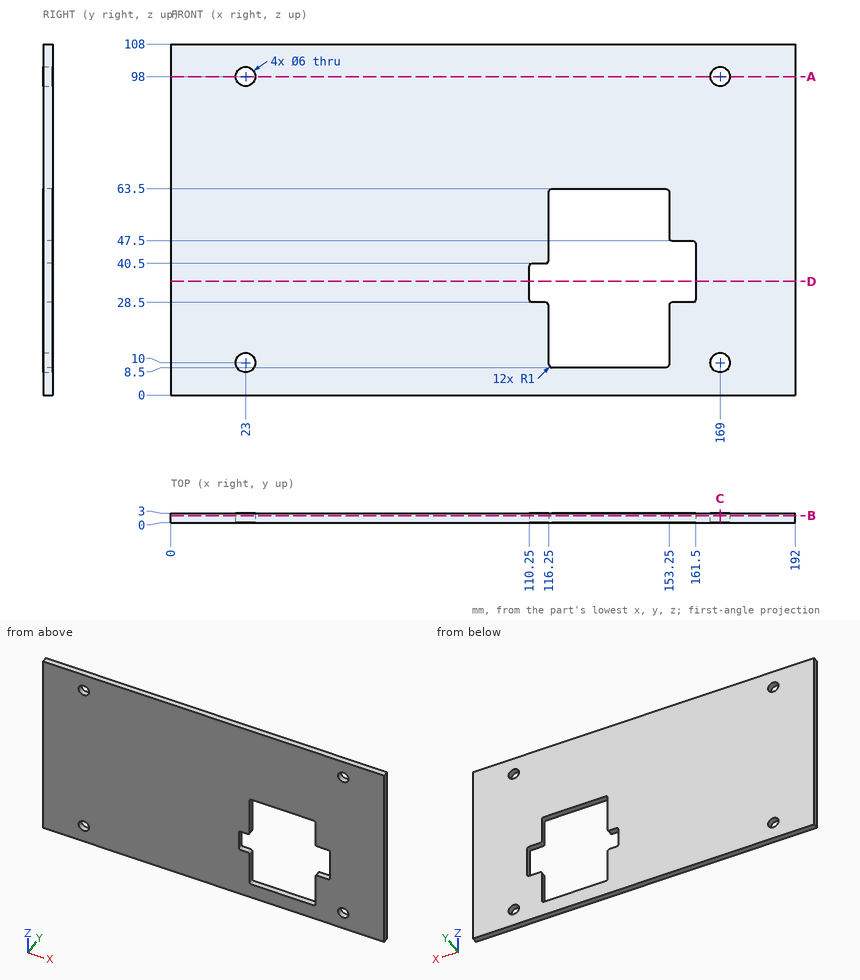
Check sheet for the drawn part. Datum: minimum x, y, z corner. Units: mm. Round coordinates to 2 decimals unless told otherwise and drop trailing zeros. Write each loop counter-clockwise with the first axis right and the second up, starting at its lowest first coordinate (ties: lowest second). Pieces come first, ordered by that corner, then holes. Notation, with made-up numbers: (-17.75, -5.5) -> (-7.75, -5.5) arc R20 cw to (-7.75, 31.5) -> close; hole circle Ø11 at (63.25, 86). An arc over 180 degrees is marked (long way). Write each question's results on one line, items separated by ' | '. Start each with the question number.
1. Material ranges on probe 1 along Z at (x, y) = (169, 2.25); probe 2 along X at (y, z) = (0.7, 98); probe 3 along X at (y, z) = (1, 10), recorded low to high. Write a range as from..to.
2. Cross-section at B-B (y = 2.25). Count the separate pieces of the cut face and the enclosed holes in it, then the cut area to 3 significant figures.
3. Cross-section at D-D (z = 35). Enter the section's corners in (x, y), then the cut area to 3 significant figures.
4. Cross-section at C-C (x = 169). Enter the section's corners in (y, z), then the cut area to 3 significant figures.
5. Depth check by flat-ended pin: P1, Ø5.5, axis at x = 23, z = 98, coming from the -Y side. Enter the tip coordinate at first touch or a pass-through.
6. Cross-section at A-A (z = 98). Enter the section's corners in (x, y), then the cut area to 3 significant figures.
Solutions:
1) probe 1: z = 0..7, 13..95, 101..108 | probe 2: x = 0..20, 26..166, 172..192 | probe 3: x = 0..20, 26..116.25, 153.25..166, 172..192
2) separate pieces: 1 | enclosed holes: 5 | area: 18,400 mm2
3) outline: (0, 0) -> (110.25, 0) -> (110.25, 3) -> (0, 3) -> close; (161.5, 0) -> (192, 0) -> (192, 3) -> (161.5, 3) -> close | area: 422 mm2
4) outline: (0, 0) -> (3, 0) -> (3, 7) -> (0, 7) -> close; (0, 13) -> (3, 13) -> (3, 95) -> (0, 95) -> close; (0, 101) -> (3, 101) -> (3, 108) -> (0, 108) -> close | area: 288 mm2
5) P1: passes through
6) outline: (0, 0) -> (20, 0) -> (20, 3) -> (0, 3) -> close; (26, 0) -> (166, 0) -> (166, 3) -> (26, 3) -> close; (172, 0) -> (192, 0) -> (192, 3) -> (172, 3) -> close | area: 540 mm2
